Can you work these out from the model? Positions are in its coordinate system, mm. A direction names the side the tool comes from. Round coordinates to 2 decimals unless told otherwise and drop trailing zeros. Loops run counter-clockwise (first coordinate to the right, second up) from the corner with the lowest first, then second, coordinate; pieces in that order, holes last. Notation, with made-up numbers: M 77,31.25 L 107,31.25 A17 cw 107,60.25 Z; hole C 35.25,-21.75 d8. An arc over 180 degrees is marked long. Answer as CSV lines item,"result".
from build123d import *

# Parameters (mm, degrees)
SKETCH1_W           = 78
SKETCH1_H           = 25
BOSS_EXTRUDE1_DEPTH = 10
SKETCH2_W           = 68
SKETCH2_H           = 15
CUT_EXTRUDE2_DEPTH  = 10
SKETCH3_W           = 25
SKETCH3_H           = 5
BOSS_EXTRUDE2_DEPTH = 10
SKETCH4_W           = 25
SKETCH4_H           = 5
BOSS_EXTRUDE3_DEPTH = 10
SKETCH6_W           = 10
SKETCH6_H           = 5
BOSS_EXTRUDE4_DEPTH = 5
SKETCH9_R           = 1.75
CUT_EXTRUDE5_DEPTH  = 2
SKETCH10_R          = 1
CUT_EXTRUDE6_DEPTH  = 13
SKETCH11_W          = 78
SKETCH11_H          = 5
CUT_EXTRUDE7_DEPTH  = 2


with BuildPart() as part:
    # Sketch1 → Boss-Extrude1 (new body)
    with BuildSketch(Plane(origin=(0, 0, 0), x_dir=(1, 0, 0), z_dir=(0, 1, 0))):
        Rectangle(SKETCH1_W, SKETCH1_H)
    extrude(amount=BOSS_EXTRUDE1_DEPTH)

    # Sketch2 → Cut-Extrude2 (cut)
    with BuildSketch(Plane(origin=(0, 10, 0), x_dir=(1, 0, 0), z_dir=(0, 1, 0))):
        Rectangle(SKETCH2_W, SKETCH2_H)
    extrude(amount=-CUT_EXTRUDE2_DEPTH, mode=Mode.SUBTRACT)

    # Sketch3 → Boss-Extrude2 (add)
    with BuildSketch(Plane.ZY.offset(39)):
        with Locations((0, 2.5)):
            Rectangle(SKETCH3_W, SKETCH3_H)
    extrude(amount=BOSS_EXTRUDE2_DEPTH)

    # Sketch4 → Boss-Extrude3 (add)
    with BuildSketch(Plane(origin=(39, 0, 0), x_dir=(0, 0, -1), z_dir=(1, 0, 0))):
        with Locations((0, 2.5)):
            Rectangle(SKETCH4_W, SKETCH4_H)
    extrude(amount=BOSS_EXTRUDE3_DEPTH)

    # Sketch6 → Boss-Extrude4 (add)
    with BuildSketch(Plane(origin=(0, 5, 0), x_dir=(1, 0, 0), z_dir=(0, 1, 0))):
        with Locations((44, 0)):
            Rectangle(SKETCH6_W, SKETCH6_H)
        with Locations((-44, 0)):
            Rectangle(SKETCH6_W, SKETCH6_H)
    extrude(amount=BOSS_EXTRUDE4_DEPTH)

    # Sketch9 → Cut-Extrude5 (cut)
    with BuildSketch(Plane.XZ):
        with Locations(Location((-44, 6.25, 0), (0, 0, 270))):
            Circle(SKETCH9_R)
        with Locations(Location((-44, -6.25, 0), (0, 0, 270))):
            Circle(SKETCH9_R)
        with Locations(Location((44, 6.25, 0), (0, 0, 270))):
            Circle(SKETCH9_R)
        with Locations(Location((44, -6.25, 0), (0, 0, 270))):
            Circle(SKETCH9_R)
    extrude(amount=-CUT_EXTRUDE5_DEPTH, mode=Mode.SUBTRACT)

    # Sketch10 → Cut-Extrude6 (cut)
    with BuildSketch(Plane.XZ.offset(-2)):
        with Locations(Location((-44, 6.25, 0), (0, 0, 270))):
            Circle(SKETCH10_R)
        with Locations(Location((-44, -6.25, 0), (0, 0, 270))):
            Circle(SKETCH10_R)
        with Locations(Location((44, 6.25, 0), (0, 0, 270))):
            Circle(SKETCH10_R)
        with Locations(Location((44, -6.25, 0), (0, 0, 270))):
            Circle(SKETCH10_R)
    extrude(amount=-CUT_EXTRUDE6_DEPTH, mode=Mode.SUBTRACT)

    # Sketch11 → Cut-Extrude7 (cut)
    with BuildSketch(Plane.XY.offset(12.5)):
        with Locations((0, 7.5)):
            Rectangle(SKETCH11_W, SKETCH11_H)
    extrude(amount=-CUT_EXTRUDE7_DEPTH, mode=Mode.SUBTRACT)


solid = part.part
Item 1: If I drill on line 1 along X through (y, z) = (1.65, 6.25); line 2 along X through (y, z) = (3.5, -6.25); line 3 along Z through (x, y) = (-28.5, 9.75), over which ranges is the centre line in solid material (lowest first)? Write a range as from..to.
Output:
line 1,"x = -49..-45.75, -42.25..-34, 34..42.25, 45.75..49"
line 2,"x = -49..-45, -43..-34, 34..43, 45..49"
line 3,"z = -12.5..-7.5, 7.5..10.5"
Item 2: If we section it at B-B on y = 7.5: Write out the boundary of the cut face in (x, z), then the cut area to 3 significant figures.
Output:
outline,"M -49,-2.5 L -39,-2.5 L -39,-12.5 L 39,-12.5 L 39,-2.5 L 49,-2.5 L 49,2.5 L 39,2.5 L 39,10.5 L -39,10.5 L -39,2.5 L -49,2.5 Z; hole M -34,-7.5 L 34,-7.5 L 34,7.5 L -34,7.5 Z"
area,"874 mm2"
Item 3: On a 3-axis mill with a long thin cutter (end or side, diameter ignored), from which of +Z, -Z, +X, -X, +Y, -Y can I reach the whole of each face in a straight line? I mean faces 4 (the face through (-39, 7, -7)), 5 (the face through (-34, 5, 0)), 6 (the face through (-45.71, 0.99, -5.87)), 7 (the face through (-44, 7, 2.5)). Say none if no direction works.
Output:
face 4,"-Z, -X, +Y"
face 5,"+Y, -Y"
face 6,"-Y"
face 7,"+Z, -X, +Y"
Item 4: If we section it at D-D on z = 6.25: Write out the boundary of the cut face in (x, y), then the cut area to 3 significant figures.
Output:
outline,"M -49,0 L -45.75,0 L -45.75,2 L -45,2 L -45,5 L -49,5 Z; M -43,2 L -42.25,2 L -42.25,0 L -34,0 L -34,10 L -39,10 L -39,5 L -43,5 Z; M 34,0 L 42.25,0 L 42.25,2 L 43,2 L 43,5 L 39,5 L 39,10 L 34,10 Z; M 45,2 L 45.75,2 L 45.75,0 L 49,0 L 49,5 L 45,5 Z"
area,"174 mm2"
Item 5: Will these pins go through, and if not, where does the flat tip stop? pin 1 (1.5 mm diameter, centred on x = -43, y = 7, fed in from -Z); pin 2 (1.5 mm diameter, centred on y = 6, z = 7, fed in from +X); pin 3 (1.6 mm diameter, centred on x = 44, z = -6.25, fed in from +Y); pin 4 (5.5 mm diameter, centred on x = 41.5, y = 7, fed in from +Z).
Output:
pin 1,"stops at z = -2.5"
pin 2,"stops at x = 39"
pin 3,"passes through"
pin 4,"stops at z = 12.5"
Item 6: If we section it at A-A on z = 0: Write out the boundary of the cut face in (x, y).
Output:
outline,"M -49,0 L -34,0 L -34,10 L -49,10 Z; M 34,0 L 49,0 L 49,10 L 34,10 Z"
Item 7: If we section it at C-C on x = 44: Write out the boundary of the cut face in (y, z), then the cut area to 3 significant figures.
Output:
outline,"M 0,-12.5 L 5,-12.5 L 5,-7.25 L 2,-7.25 L 2,-8 L 0,-8 Z; M 0,-4.5 L 2,-4.5 L 2,-5.25 L 5,-5.25 L 5,-2.5 L 10,-2.5 L 10,2.5 L 5,2.5 L 5,5.25 L 2,5.25 L 2,4.5 L 0,4.5 Z; M 0,8 L 2,8 L 2,7.25 L 5,7.25 L 5,12.5 L 0,12.5 Z"
area,"124 mm2"
Item 8: We'd pull the mould along Z, two halves only. Please class faces 1 (the face through (44, 7, -2.5)), 2 (the face through (42.29, 0.99, 6.63)), 3 (the face through (-1, 0, 9)): released by +Z, released by -Z, zero draft, split by the parting line, or undercut.
Output:
face 1,"released by -Z"
face 2,"undercut"
face 3,"zero draft"
